Work out the finished part from the listing and answer in its coordinate system (mm). A direction names the side the tool comes from. Coordinates: 2 decimals unless noted, no trailing zeros. Order: outer loops, then holes, each group sorted by start corner. A loop starts at its lowest first (then second) coordinate and runs counter-clockwise, first axis right, second up. Notation, with made-up numbers: (46.5, -5.75) - (56.5, -5.75) arc R11 ccw to (56.5, 8.25) - close; hole circle Ø2 at (6, 5.5). An arc over 180 degrees is marked (long way). Answer as a JSON object with one key per item and string values. Group by question number.
1) Section A-A (x = -31) is taken. Give the vertices of the cut face in (y, z), plus the area to 3 significant figures.
2) Section B-B (x = -16) is taken. Give the vertices of the cut face in (y, z).
3) Each of these flat-tipped pins is pushed along its axis until it touches: P1, Ø5.5, axis at x = -28.02, y = 29.25, coming from the +Z side; P2, Ø10.5, axis at x = -64.99, y = 38.47, coming from the -Z side; P3, Ø10, axis at x = -44.5, y = 56.5, coming from the +Z side; P4, Ø1.5, axis at x = -59, y = 18.5, coming from the +Z side. Where does it stop, or does it pass through?
4) The mould has two halves that part along Y. Classify faces 1 (the face through (-80.301, 45.497, 6.505)), 2 (the face through (-46, 38, 0)), 3 (the face through (-46, 0, 14)), 4 (the face through (-67.99, 32.7, 9.09)): released by +Y, released by -Y, zero draft, split by the parting line, or undercut.
5) Find the intervals of material crossed by line 1 along X through (y, z) = (28.5, 5.75); line 2 along Z through (x, y) = (-70.5, 38); line 3 along X through (y, z) = (35, 9.75), in increasing order.
6) A tool of negligible diameter and unlimited length cuts with its end or side. For faces 5 (the face through (-46, 62.79, 2)), 6 (the face through (-26, 25, 4.69)), 7 (the face through (-20.301, 17.306, 16.766)), from which of +Z, -Z, +X, -X, +Y, -Y can it reach the whole face along a straight path? Write none if from no direction.
7) Section D-D (x = -54) is taken. Give the vertices of the cut face in (y, z), plus the area to 3 significant figures.
8) Section C-C (y = 46.5) is taken. Count the separate pieces of the cut face and the enclosed holes in it, plus the area to 3 significant figures.
from build123d import *

# Parameters (mm, degrees)
BOSS_EXTRUDE1_DEPTH = 94.24
SKETCH2_R           = 4.5
CUT_EXTRUDE1_DEPTH  = 94.24
CUT_EXTRUDE2_START  = -4.69
SKETCH2_3_R         = 6.5
CUT_EXTRUDE2_DEPTH  = 94.24
SKETCH3_R           = 3
CUT_EXTRUDE3_DEPTH  = 94.24
CUT_EXTRUDE4_START  = -4.5
SKETCH3_3_R         = 4.75
CUT_EXTRUDE4_DEPTH  = 94.24


with BuildPart() as part:
    # Sketch1 → Boss-Extrude1 (new body)
    with BuildSketch(Plane(origin=(0, 0, 0), x_dir=(0, 0, -1), z_dir=(1, 0, 0))):
        Polygon((0, 0), (0, 62.78974436), (-5, 62.78974436), (-27.85359797, 0), align=None)
    extrude(amount=-BOSS_EXTRUDE1_DEPTH)

    # Sketch2 → Cut-Extrude1 (cut)
    with BuildSketch(Plane(origin=(0, 0, 0), x_dir=(-1, 0, 0), z_dir=(0, 0, -1))):
        with Locations((28.02184799, 29.25081122)):
            Circle(SKETCH2_R)
        with Locations((64.99011516, 38.46803544)):
            Circle(SKETCH2_R)
    extrude(amount=-CUT_EXTRUDE1_DEPTH, mode=Mode.SUBTRACT)

    # Sketch2_3 → Cut-Extrude2 (cut)
    with BuildSketch(Plane(origin=(0, 0, 0), x_dir=(-1, 0, 0), z_dir=(0, 0, -1)).offset(CUT_EXTRUDE2_START)):
        with Locations((28.02184799, 29.25081122)):
            Circle(SKETCH2_3_R)
        with Locations((64.99011516, 38.46803544)):
            Circle(SKETCH2_3_R)
    extrude(amount=-CUT_EXTRUDE2_DEPTH, mode=Mode.SUBTRACT)

    # Sketch3 → Cut-Extrude3 (cut)
    with BuildSketch(Plane(origin=(0, 8.951973832, 24.595345956), x_dir=(1, 0, 0), z_dir=(0, 0.3420201434019967, 0.9396926207581273))):
        with Locations(Location((-17.20092637, 11.517541778, 0), (0, 0, 270))):
            Circle(SKETCH3_R)
        with Locations(Location((-17.20092637, 41.517541778, 0), (0, 0, 270))):
            Circle(SKETCH3_R)
        with Locations(Location((-47.20092637, 26.517541778, 0), (0, 0, 270))):
            Circle(SKETCH3_R)
        with Locations(Location((-77.20092637, 41.517541778, 0), (0, 0, 270))):
            Circle(SKETCH3_R)
        with Locations(Location((-77.20092637, 11.517541778, 0), (0, 0, 270))):
            Circle(SKETCH3_R)
    extrude(amount=-CUT_EXTRUDE3_DEPTH, mode=Mode.SUBTRACT)

    # Sketch3_3 → Cut-Extrude4 (cut)
    with BuildSketch(Plane(origin=(0, 8.951973832, 24.595345956), x_dir=(1, 0, 0), z_dir=(0, 0.3420201434019967, 0.9396926207581273)).offset(CUT_EXTRUDE4_START)):
        with Locations(Location((-17.20092637, 11.517541778, 0), (0, 0, 270))):
            Circle(SKETCH3_3_R)
        with Locations(Location((-17.20092637, 41.517541778, 0), (0, 0, 270))):
            Circle(SKETCH3_3_R)
        with Locations(Location((-47.20092637, 26.517541778, 0), (0, 0, 270))):
            Circle(SKETCH3_3_R)
        with Locations(Location((-77.20092637, 11.517541778, 0), (0, 0, 270))):
            Circle(SKETCH3_3_R)
        with Locations(Location((-77.20092637, 41.517541778, 0), (0, 0, 270))):
            Circle(SKETCH3_3_R)
    extrude(amount=-CUT_EXTRUDE4_DEPTH, mode=Mode.SUBTRACT)


solid = part.part
Report:
{
 "1": {"outline": "(0, 0) - (25.88, 0) - (25.88, 4.69) - (23.47, 4.69) - (23.47, 19.31) - (0, 27.85) - close; (32.62, 0) - (62.79, 0) - (62.79, 5) - (35.03, 15.1) - (35.03, 4.69) - (32.62, 4.69) - close", "area": "855 mm²"},
 "2": {"outline": "(0, 0) - (7.37, 0) - (13.92, 18) - (15.65, 17.37) - (17.19, 21.6) - (0, 27.85) - close; (17.15, 0) - (39.29, 0) - (42.11, 7.74) - (43.84, 7.11) - (45.38, 11.34) - (22.36, 19.72) - (20.82, 15.49) - (22.55, 14.86) - close; (49.01, 5.23) - (50.75, 4.6) - (49.07, 0) - (62.79, 0) - (62.79, 5) - (50.55, 9.46) - close"},
 "3": {"P1": "passes through", "P2": "stops at z = 0", "P3": "stops at z = 9.11", "P4": "stops at z = 21.39"},
 "4": {"face 1": "undercut", "face 2": "zero draft", "face 3": "released by -Y", "face 4": "undercut"},
 "5": {"line 1": "x = -94.24 to -51.64, -42.77 to -34.48, -21.57 to 0", "line 2": "z = 0 to 4.69", "line 3": "x = -94.24 to -70.49, -59.49 to -50.85, -43.55 to -31.05, -24.99 to 0"},
 "6": {"face 5": "+Z, -Z, +X, -X, +Y", "face 6": "+Z", "face 7": "none"},
 "7": {"outline": "(0, 0) - (62.79, 0) - (62.79, 5) - (0, 27.85) - close", "area": "1,030 mm²"},
 "8": {"separate pieces": "3", "enclosed holes": "0", "area": "863 mm²"}
}
